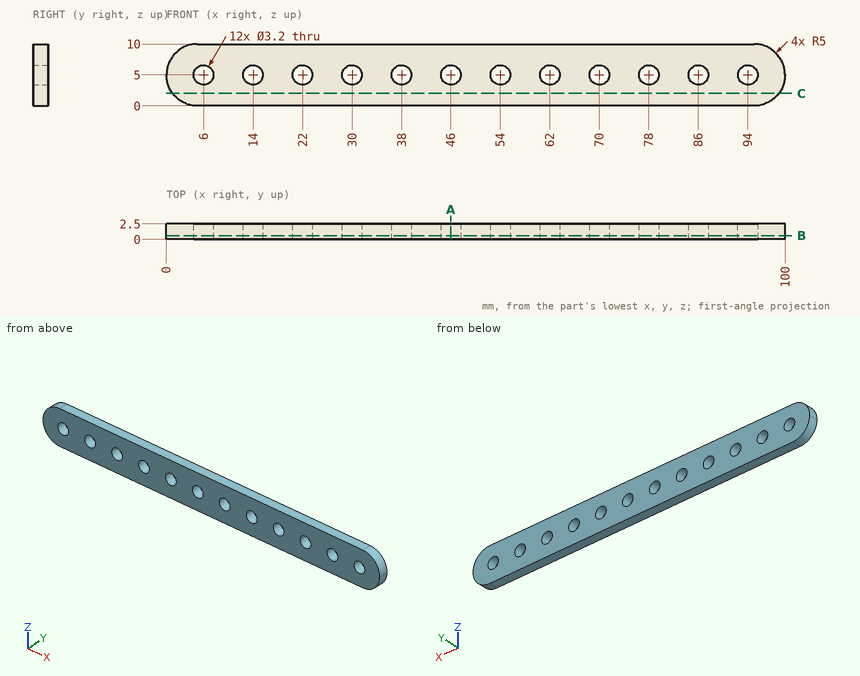
The drawing under review shows one solid part. Ordinate dimensions are in mm from its lowest x, y, z. Coordinates: 2 decimals unless noted, no trailing zeros. Loops run counter-clockwise (first coordinate to the right, second up) from the corner with the lowest first, then second, coordinate; pieces in that order, holes last. Notation, with made-up numbers: M 77.5,-20 L 126.5,-20 A16 ccw 126.5,-5 Z; hole C -23,-8 d7. An arc over 180 degrees is marked long. Use one line per item in the form item = value.
(1) For line 1 along Z through (x, y) = (70, 1.5); line 2 along Z through (x, y) = (21, 0.9); line 3 along X through (y, z) = (1.95, 2), list the stretches that pass through material, from the lowest coordinate up. Write a range as from..to.
Return value:
line_1 = 0..3.4, 6.6..10
line_2 = 0..3.75, 6.25..10
line_3 = 1..99
(2) Consider section B-B (y = 0.6). Give the number of separate pieces and of enclosed holes in the cut face, and give its area (3 significant figures).
Return value:
separate_pieces = 1
enclosed_holes = 12
area = 882 mm2
(3) Clearance check with flat-ended pins moving along their axes: P1, Ø2.5, axis at x = 6, z = 5, coming from the +Y side; P2, Ø1, axis at y = 1, z = 2, coming from the +X side. State where each tip first meets the part, or that it passes through.
Return value:
P1 = through
P2 = 99.33
(4) Consider section A-A (x = 46). Write out the cut boundary in (y, z).
Return value:
outline = M 0,0 L 2.5,0 L 2.5,3.4 L 0,3.4 Z; M 0,6.6 L 2.5,6.6 L 2.5,10 L 0,10 Z
(5) Consider section C-C (z = 2). Write out the cut boundary in (x, y), and give its area (3 significant figures).
Return value:
outline = M 1,0 L 99,0 L 99,2.5 L 1,2.5 Z
area = 245 mm2
